Here's how the part is built. I have some questions about the finished solid (model axes, mm). A direction names the side the tool comes from. Round coordinates to 2 decimals unless told otherwise and drop trailing zeros. Write each loop counter-clockwise with the first axis right and the second up, starting at its lowest first coordinate (ties: lowest second). Pieces come first, ordered by that corner, then holes. Notation, with made-up numbers: (11.5, -33.5) - (70.5, -33.5) arc R5 cw to (70.5, -25.5) - close; hole circle Ø4 at (27, -3). An arc over 180 degrees is marked (long way). One line per item, written item: value. Start each with the question number.
Item 1: Thinking about a two-plate mould opening in X: for faces 1 (the face through (-170.435, 96.265, 219.289)), 2 (the face through (-149.225, 80, 146)), 3 (the face through (-1, 40, 0)), 4 (the face through (-186.79, 19.35, 292.6)), which applies, released by +X, released by -X, zero draft, split by the parting line, or undercut?
Item 2: For faces 5 (the face through (-2, 41.275, 66)), 6 (the face through (-2, -38.1, 75)), 7 (the face through (-189.413, 19.35, 290.117)), which set-ups out of +Z, -Z, +X, -X, +Y, -Y let a thin tool reach every point of the face, with its end or its side?
Item 3: For P1, Ø1.4, axis at y = 43, z = 143, coming from the +X side (3 decimals); P2, Ø3, axis at x = -121.5, z = 197, coming from the +Y side; P3, Ø9.5, axis at x = -193, z = 142, coming from the -Y side (3 decimals), each with a flat end and sliding along its axis, tell me the tip position at first contact or that it passes through.
Item 4: Imagine slicing it at B-B, the plane z = 66.5. Please give me the cut outline in (x, y) (3 decimals), then the cut area to 3 significant figures.
Item 5: Imagine slicing it at A-A, the plane x = 80. Please give me the cut outline in (y, z) (3 decimals), then the cut area to 3 significant figures.
Item 6: If I drill on line 1 (Y direction, x = 5.5, z = 126) (3 decimals); line 2 (X direction, y = -18, z = 122) (3 decimals); line 3 (X direction, y = 32, z = 163.5), over which ranges is the centre line in solid material (lowest first)?
Item 7: Imagine slicing it at C-C, the plane y = 15. Please give me the cut outline in (x, z) (3 decimals).
Item 8: Imagine slicing it at D-D, the plane y = 64. Please give me the cut outline in (x, z) (3 decimals), then the cut area to 3 significant figures.
```python
from build123d import *

# Parameters (mm, degrees)
F0_W          = 298.45
F0_H          = 82.55
F0_W_2        = 292.1
F0_H_2        = 76.2
F1_DEPTH      = 152.4
F4_DEPTH      = 158.75
F5_DEPTH      = 254
F5_DEPTH_BACK = 76.2
F7_DEPTH      = 25.4


with BuildPart() as f1:
    # F0 (on Top) → F1 (new body)
    with BuildSketch(Plane.XY):
        Rectangle(F0_W, F0_H)
        Rectangle(F0_W_2, F0_H_2, mode=Mode.SUBTRACT)
    extrude(amount=F1_DEPTH)

    # F2 (on face) → F4 (join)
    with BuildSketch(Plane.XZ.offset(41.275)):
        Polygon((-149.225, 140.1327420061), (-149.225, 152.4), (-225.425, 436.7822715367), (-228.4918144985, 435.9605210685), align=None)
    extrude(amount=-F4_DEPTH)

    # F3 (on face) → F5 (join, two sides)
    with BuildSketch(Plane(origin=(-149.225, 0, 0), x_dir=(0, -1, 0), z_dir=(-1, 0, 0))) as f5_sk:
        Polygon((-41.275, 133.7086633322), (-41.275, 152.4), (-117.475, 436.7822715367), (-122.147834167, 435.5301893953), align=None)
    extrude(amount=-F5_DEPTH)
    extrude(f5_sk.sketch, amount=F5_DEPTH_BACK)

    # F6: F1 across plane


with BuildPart() as f1_1:
    add(f1.part)
    add(f1.part.mirror(Plane.YZ))

    # F7 (cut): a face of the model
    f7_faces = [f1_1.faces().sort_by_distance(p)[0] for p in [
        (201.1206672909, 65.5793327091, 243.1050045143),
    ]]
    extrude(f7_faces, amount=-F7_DEPTH, mode=Mode.SUBTRACT)


solid = f1_1.part
```
Values follow:
1. face 1: released by -X
1. face 2: undercut
1. face 3: zero draft
1. face 4: undercut
2. face 5: -Z, +X, -X, +Y
2. face 6: +Z, -Z
2. face 7: -X, -Y
3. P1: stops at x = 225.425
3. P2: stops at y = 58.64
3. P3: stops at y = 41.275
4. outline: (-149.225, -41.275) - (149.225, -41.275) - (149.225, 41.275) - (-149.225, 41.275) - close; hole (-146.05, -38.1) - (146.05, -38.1) - (146.05, 38.1) - (-146.05, 38.1) - close
4. area: 2,380 mm^2
5. outline: (-41.275, 0) - (-38.1, 0) - (-38.1, 152.4) - (-41.275, 152.4) - close; (38.1, 0) - (41.275, 0) - (41.275, 133.709) - (122.148, 435.53) - (117.475, 436.782) - (41.275, 152.4) - (38.1, 152.4) - close
5. area: 2,440 mm^2
6. line 1: y = -41.275 to -38.1, 38.1 to 41.275
6. line 2: x = -149.225 to -146.05, 146.05 to 149.225
6. line 3: x = -155.49 to -152.2, 152.2 to 155.49
7. outline: (-228.492, 435.961) - (-149.225, 140.133) - (-149.225, 0) - (-146.05, 0) - (-146.05, 152.4) - (-149.225, 152.4) - (-225.425, 436.782) - close; (146.05, 0) - (149.225, 0) - (149.225, 140.133) - (228.492, 435.961) - (225.425, 436.782) - (149.225, 152.4) - (146.05, 152.4) - close
8. outline: (-228.492, 435.961) - (-175.237, 237.211) - (-225.425, 237.211) - (-225.425, 218.52) - (-170.229, 218.52) - (-149.225, 140.133) - (-149.225, 152.4) - (-166.942, 218.52) - (166.942, 218.52) - (149.225, 152.4) - (149.225, 140.133) - (170.229, 218.52) - (170.564, 218.52) - (175.237, 237.211) - (228.492, 435.961) - (225.425, 436.782) - (171.95, 237.211) - (-171.95, 237.211) - (-225.425, 436.782) - close
8. area: 9,230 mm^2
